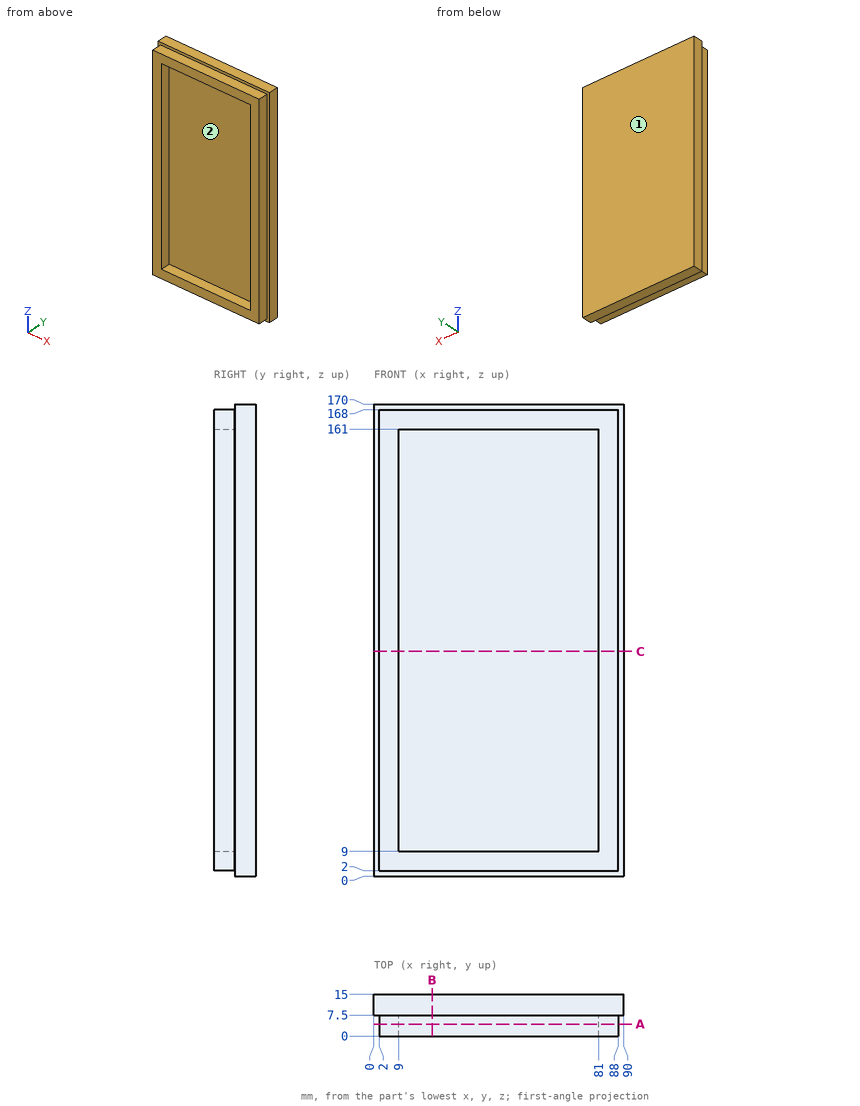
Part print with two shaded views. Sizes in mm from the minimum x, y, z corner. Give positions to 0.01 mm unless a question says otherwise; leave off trailing zeros. Order: outer loops, then holes, each group sorted by start corner. A loop starts at its lowest first (then second) coordinate and runs counter-clockwise, first axis right, second up.
(1) Saw through at C-C, the plane z = 81. Give the cut face in (x, y).
(2) Mould opens along Z. For the marked faces 1 and 2 say: released by +Z, released by -Z, zero draft, split by the parting line, or undercut.
(3) Flat gauge pins, fed straight in: pin 1 (8 mm diameter, centred on x = 72, z = 113, fed in from -Y); pin 2 (2 mm diameter, centred on x = 66.5, y = 5, fed in from -Z); pin 3 (4 mm diameter, centred on y = 2.5, z = 85.5, fed in from +X). Where does each tip first touch, or does it go through?
(4) Saw through at A-A, the plane y = 4.25. Give the cut face in (x, z).
(5) Drill centre lines: L1, parallel to X at y = 7, z = 30.5; L2, parallel to Z at x = 73, y = 7; L3, parallel to Y at x = 64.5, z = 125. Where is each one in solid material? Low to high.
(6) Saw through at B-B, the plane x = 21. Give the cut face in (y, z).
Results found:
1. outline: (0, 7.5) - (2, 7.5) - (2, 0) - (9, 0) - (9, 7.5) - (81, 7.5) - (81, 0) - (88, 0) - (88, 7.5) - (90, 7.5) - (90, 15) - (0, 15) - close
2. face 1: zero draft
2. face 2: undercut
3. pin 1: stops at y = 7.5
3. pin 2: stops at z = 2
3. pin 3: stops at x = 88
4. outline: (2, 2) - (88, 2) - (88, 168) - (2, 168) - close; hole (9, 9) - (81, 9) - (81, 161) - (9, 161) - close
5. L1: x = 2 to 9, 81 to 88
5. L2: z = 2 to 9, 161 to 168
5. L3: y = 7.5 to 15
6. outline: (0, 2) - (7.5, 2) - (7.5, 0) - (15, 0) - (15, 170) - (7.5, 170) - (7.5, 168) - (0, 168) - (0, 161) - (7.5, 161) - (7.5, 9) - (0, 9) - close
